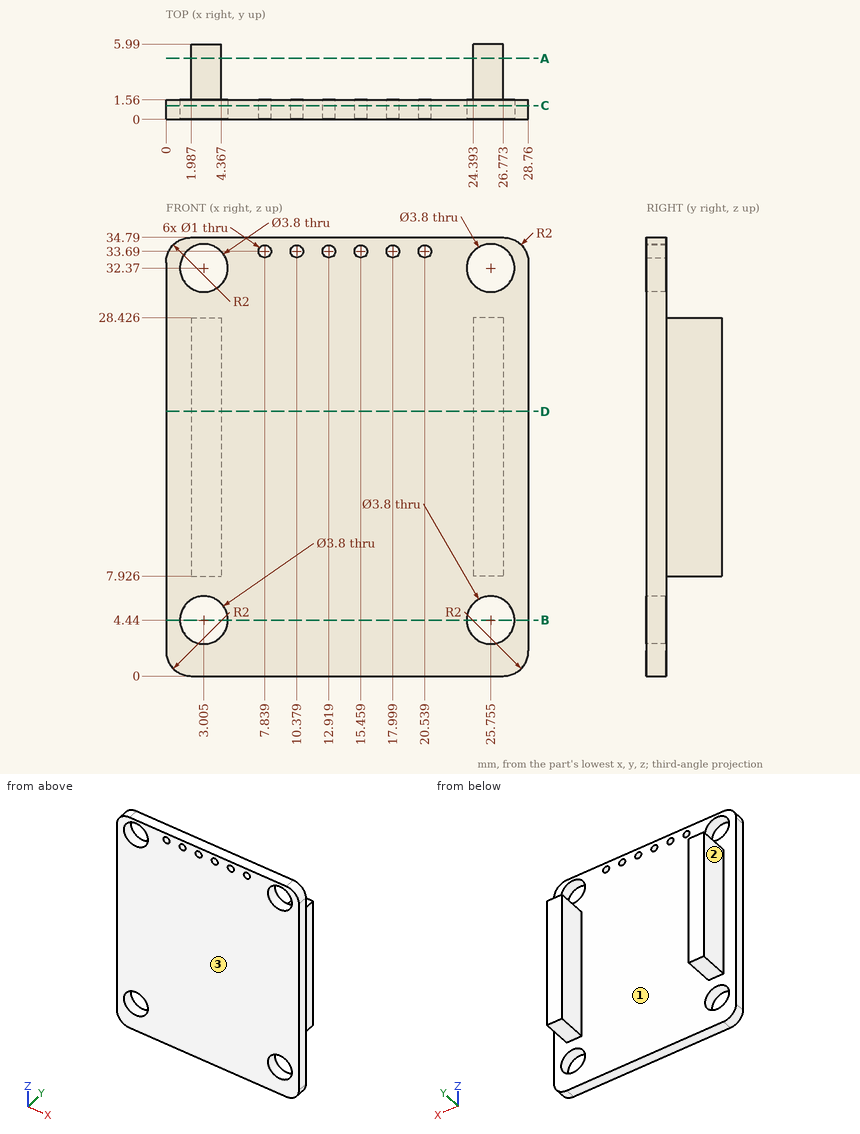
Check sheet for the drawn part. Datum: minimum x, y, z corner. Units: mm. Round coordinates to 2 decimals unless told otherwise and drop trailing zeros. Order: outer loops, then holes, each group sorted by start corner. A loop starts at its lowest first (then second) coordinate and runs counter-clockwise, first axis right, second up. Notation, with made-up numbers: M -15,37 L 19,37 A24 cw 19,64 Z; hole C 87.25,30 d3. An arc over 180 degrees is marked long. Answer in a Markdown table with one row per item.
(1) Section check A-A on y = 4.85. Record the boundary of the cut face in (x, z).
Findings:
| item | result |
|---|---|
| outline | M 1.99,7.93 L 4.37,7.93 L 4.37,28.43 L 1.99,28.43 Z; M 24.39,7.93 L 26.77,7.93 L 26.77,28.43 L 24.39,28.43 Z |
(2) Draft check along X on the marked faces 1, 2 and 3. Enter one of: +X half, -X half, draft (parallel to the pull), parting line (faces both ways), or undercut.
Findings:
| item | result |
|---|---|
| face 1 | undercut |
| face 2 | -X half |
| face 3 | draft |
(3) Material ranges on line 1 along X through (y, z) = (1.2, 4.44) (1 decimal); line 2 along Z through (x, y) = (25.75, 0.65); line 3 along X through (y, z) = (1.6, 13), recorded low to high. Write a range as from..to.
Findings:
| item | result |
|---|---|
| line 1 | x = 0..1.1, 4.9..23.9, 27.7..28.8 |
| line 2 | z = 0..2.54, 6.34..30.47, 34.27..34.79 |
| line 3 | x = 1.99..4.37, 24.39..26.77 |
(4) Section check B-B on z = 4.44. Record the boundary of the cut face in (x, y) (1 decimal).
Findings:
| item | result |
|---|---|
| outline | M 0,0 L 1.1,0 L 1.1,1.6 L 0,1.6 Z; M 4.9,0 L 23.9,0 L 23.9,1.6 L 4.9,1.6 Z; M 27.7,0 L 28.8,0 L 28.8,1.6 L 27.7,1.6 Z |
(5) Gauge pin test, flat ends, axial feed: pin 1 (3 mm diameter, centred on x = 5, z = 5.5, fed in from +Y); pin 2 (2.5 mm diameter, centred on x = 3, y = 5, fed in from -Z); pin 3 (1.9 mm diameter, centred on x = 26, y = 3, fed in from +Z); pin 4 (2.5 mm diameter, centred on x = 25.755, z = 4.44, fed in from +Y). Record the tip position at first contact, or that the pin passes through.
Findings:
| item | result |
|---|---|
| pin 1 | stops at y = 1.56 |
| pin 2 | stops at z = 7.93 |
| pin 3 | stops at z = 28.43 |
| pin 4 | passes through |
(6) Section check D-D on z = 21. Record the boundary of the cut face in (x, y).
Findings:
| item | result |
|---|---|
| outline | M 0,0 L 28.76,0 L 28.76,1.56 L 26.77,1.56 L 26.77,5.99 L 24.39,5.99 L 24.39,1.56 L 4.37,1.56 L 4.37,5.99 L 1.99,5.99 L 1.99,1.56 L 0,1.56 Z |
(7) Section check C-C on y = 1.1. Give the number of separate pieces and of enclosed holes in the cut face, plus the area to 3 significant figures.
Findings:
| item | result |
|---|---|
| separate pieces | 1 |
| enclosed holes | 10 |
| area | 947 mm^2 |
